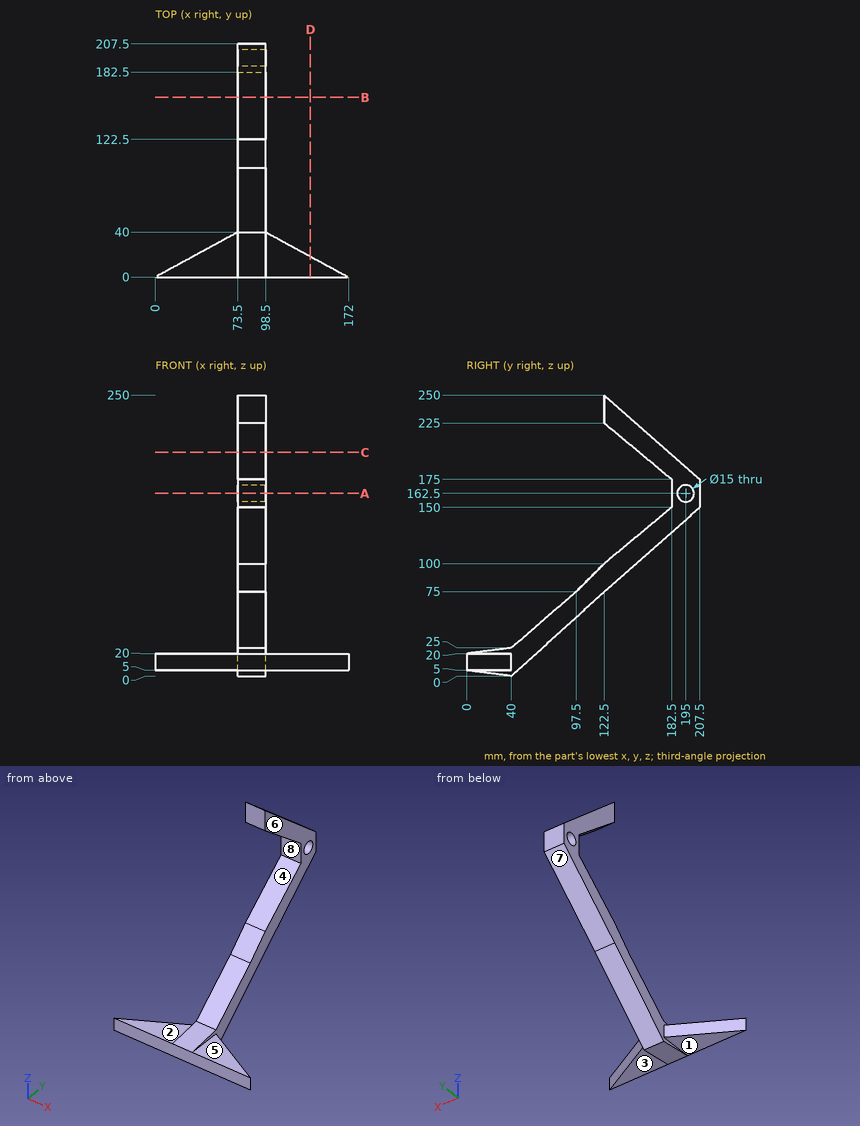
Answer from the drawing. Dimensions are ordinates in mm from the lowest x, y and z of the part. A direction names the side the tool comes from. Round coordinates to 2 decimals unless told otherwise and drop trailing zeros. Order: outer loops, then holes, each group sorted by start corner. A loop starts at its lowest first (then second) coordinate and runs counter-clockwise, first axis right, second up.
1) The mould has two halves that part along Z. Classify the marked faces 5, 6, 7 and 8: released by +Z, released by -Z, zero draft, split by the parting line, or undercut.
2) For the marked faces 1, 2, 3 and 4, determine the directions among +Z, -Z, +X, -X, +Y, -Y from which every point of the face is accessible in a straight line to the end or side of a thin tool.
3) The part is cut by section A-A on z = 162.5. Write down the section's boundary in (x, y).
4) The part is cut by section B-B on y = 160. Write down the section's boundary in (x, z), plus the area to 3 significant figures.
5) Straight lines are drawn through the part: L1, parallel to Y at x = 80.25, z = 162.5; L2, parallel to Z at x = 41, y = 12.5; L3, parallel to X at y = 192, z = 138. For each, find the intervals that lie inside material, in ascending order.
6) The part is cut by section C-C on z = 199. Write down the section's boundary in (x, y), plus the area to 3 significant figures.
7) Flat-ended cylindrical pins translate along their axes: pin 1 (5 mm diameter, centred on y = 75, z = 46, fed in from +X); pin 2 (10 mm diameter, centred on x = 85, z = 153, fed in from -Y); pin 3 (20 mm diameter, centred on x = 19.5, y = 10.5, fed in from +Z). Find the tip coordinate at first contact, or state that the pin passes through.
8) The part is cut by section D-D on x = 138. Write down the section's boundary in (y, z), plus the area to 3 significant figures.
Resolved:
1. face 5: released by +Z
1. face 6: zero draft
1. face 7: released by -Z
1. face 8: undercut
2. face 1: -Z, -X, +Y, -Y
2. face 2: +Z, -X, +Y, -Y
2. face 3: -Z, +X, +Y, -Y
2. face 4: +X, -X, -Y
3. outline: (73.5, 182.5) - (98.5, 182.5) - (98.5, 187.5) - (73.5, 187.5) - close; (73.5, 202.5) - (98.5, 202.5) - (98.5, 207.5) - (73.5, 207.5) - close
4. outline: (73.5, 108.09) - (98.5, 108.09) - (98.5, 131.25) - (73.5, 131.25) - close; (73.5, 193.75) - (98.5, 193.75) - (98.5, 216.91) - (73.5, 216.91) - close
4. area: 1,160 mm2
5. L1: y = 182.5 to 187.5, 202.5 to 207.5
5. L2: z = 5 to 20
5. L3: x = 73.5 to 98.5
6. outline: (73.5, 153.7) - (98.5, 153.7) - (98.5, 180.3) - (73.5, 180.3) - close
6. area: 665 mm2
7. pin 1: stops at x = 98.5
7. pin 2: stops at y = 180.1
7. pin 3: stops at z = 20
8. outline: (0, 5) - (18.5, 5) - (18.5, 20) - (0, 20) - close
8. area: 278 mm2
